Build history of the part. All positions in model axes, mm. Face numbers are marked on the shaded views. A direction names the side the tool comes from. Round coordinates to 2 decimals unless told otherwise and drop trailing zeros. Order: outer loops, then holes, each group sorted by start corner. A loop starts at its lowest first (then second) coordinate and runs counter-clockwise, first axis right, second up. Notation, with made-up numbers: (19, -2.75) -> (71, -2.75) arc R6 ccw to (71, 2.25) -> close; hole circle Ø6 at (-34.5, 25). An arc over 180 degrees is marked (long way). Use a Markdown table: item, result. Add a question column.
Item 1: 3-axis set-ups, long thin cutter, end or side, ignore diameter. For the marked faces 4, 5 and 6: which of +Z, -Z, +X, -X, +Y, -Y reach the whole face in a straight line?
Item 2: Slice it at D-D, the plane x = 10. Give the cut face in (y, z).
Item 3: Probe L1, parallel to Y at x = 10, z = 1.2; L2, parallel to X at y = -3, z = -3.88; L3, parallel to X at y = -7.5, z = -4.5. List the from-to ranges inside material, lowest first.
Item 4: Pin check, flat tips, straight feed: pin 1 (4.5 mm diameter, centred on x = 10, y = -8, fed in from +Z); pin 2 (1.6 mm diameter, centred on x = 24, z = -3.5, fed in from +Y); pin 3 (1 mm diameter, centred on x = 24.5, z = -4.5, fed in from -Y); pin 4 (2 mm diameter, centred on y = -6.5, z = -2, fed in from -X). Stop position of each tip, or through.
Item 5: Slice it at C-C, the plane y = -8. Give the cut face in (x, z), plus the area to 3 significant figures.
Item 6: Slice it at A-A, the plane x = 25. Give the cut face in (y, z).
Item 7: Slice it at B-B, the plane z = -3.88. Give the cut face in (x, y).
Item 8: Two-plate mould, pull along X, no slides. Class the marked faces 1, 2 and 3: released by +X, released by -X, zero draft, split by the parting line, or undercut.
Autodesk Inventor part; units mm, degrees
ref_plane "YZ Plane" through (0, 0, 0) normal (1, 0, 0) x (0, 1, 0)
ref_plane "XZ Plane" through (0, 0, 0) normal (0, 1, 0) x (-1, 0, 0)
ref_plane "XY Plane" through (0, 0, 0) normal (0, 0, 1) x (1, 0, 0)
sketch "Sketch1" plane through (0, 0, 0) normal (0, 0, 1) x (1, 0, 0)
  line L0 (0, 0) -> (20, 0)
  line L1 (20, 0) -> (20, -16)
  line L2 (20, -16) -> (0, -16)
  line L3 (0, -16) -> (0, 0)
  circle A0 centre (10, -8) radius 2.5
  dimension "d0" = 20
  dimension "d1" = 16
  dimension "d2" = 8
  dimension "d3" = 10
  dimension "d4" = 5
extrude "Extrusion1" add sketch "Sketch1" along normal blind 5
sketch "Sketch2" plane through (0, 0, 0) normal (0, 1, 0) x (1, 0, 0)
  line L0 (20, 0) -> (20, -5)
  line L1 (20, 0) -> (30, 0)
  line L2 (30, 0) -> (30, 7)
  line L3 (30, 7) -> (20, 7)
  line L4 (20, 7) -> (20, 0)
  line L5 (20, -5) -> (30, -5)
  line L6 (30, -5) -> (30, 0)
  line L7 (30, 0) -> (20, 0)
  line L8 (20, 0) -> (20, -5)
  circle A0 centre (25, 3.88) radius 2.6
  point P0 (0, 0)
  dimension "d7" = 10
  dimension "d8" = 7
  dimension "d9" = 5.2
extrude "Extrusion2" add sketch "Sketch2" against normal blind 16
sketch "Sketch3" plane through (0, -16, 0) normal (0, -1, 0) x (1, 0, 0)
  line L0 (30, -7) -> (30, 5)
  line L1 (0, 0) -> (20, 0)
  line L2 (30, -7) -> (20, -7)
  line L3 (20, -7) -> (20, 0)
  line L4 (20, 0) -> (30, 0)
  line L5 (30, 0) -> (30, -7)
extrude "Extrusion3" add sketch "Sketch3" against normal blind 9
sketch "Sketch4" plane through (0, -16, 0) normal (0, -1, 0) x (1, 0, 0)
  circle A0 centre (25, -3.88) radius 2.6
  circle A1 centre (25, -3.88) radius 2.6
  point P0 (0, 0)
  dimension "d16" = 5.2
extrude "Extrusion4" cut sketch "Sketch4" against normal blind 5
properties part number "cover mount LR v03"
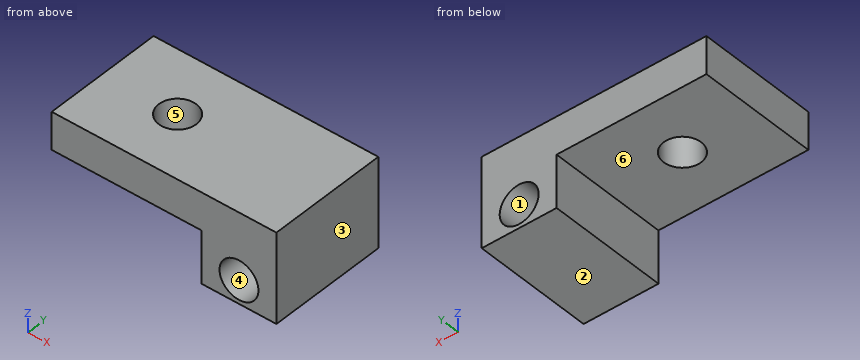
Check sheet entries:
| question | item | result |
|---|---|---|
| 1 | face 4 | -Y |
| 1 | face 5 | +Z, -Z |
| 1 | face 6 | -Z, -X, +Y, -Y |
| 2 | outline | (-16, 0) -> (-10.5, 0) -> (-10.5, 5) -> (-16, 5) -> close; (-5.5, 0) -> (0, 0) -> (0, 5) -> (-5.5, 5) -> close |
| 3 | L1 | -16 to -10.5, -5.5 to 0 |
| 3 | L2 | 20 to 22.4, 27.6 to 30 |
| 3 | L3 | 20 to 30 |
| 4 | pin 1 | through |
| 4 | pin 2 | y = -7 |
| 4 | pin 3 | y = -11 |
| 4 | pin 4 | x = 20 |
| 5 | outline | (0, 0) -> (7.5, 0) -> (7.5, 5) -> (0, 5) -> close; (12.5, 0) -> (20, 0) -> (20, -7) -> (30, -7) -> (30, 5) -> (12.5, 5) -> close |
| 5 | area | 195 mm2 |
| 6 | outline | (-16, -7) -> (0, -7) -> (0, -6.48) -> (-7, -6.48) -> (-7, -1.28) -> (0, -1.28) -> (0, 5) -> (-16, 5) -> (-16, -1.28) -> (-11, -1.28) -> (-11, -6.48) -> (-16, -6.48) -> close |
| 7 | outline | (20, -16) -> (22.4, -16) -> (22.4, -11) -> (27.6, -11) -> (27.6, -16) -> (30, -16) -> (30, 0) -> (27.6, 0) -> (27.6, -7) -> (22.4, -7) -> (22.4, 0) -> (20, 0) -> close |
| 8 | face 1 | undercut |
| 8 | face 2 | zero draft |
| 8 | face 3 | released by +X |
